Part print with two shaded views. Sizes in mm from the minimum x, y, z corner. A direction names the side the tool comes from. Coordinates: 2 decimals unless noted, no trailing zeros. Order: outer loops, then holes, each group sorted by start corner. A loop starts at its lowest first (then second) coordinate and runs counter-clockwise, first axis right, second up. Notation, with made-up numbers: M -18.5,3.5 L 16.5,3.5 A15 ccw 16.5,32.5 Z; hole C 63.25,20 d7. An arc over 180 degrees is marked long. Answer in a Markdown table with one row per item. Add a question column.
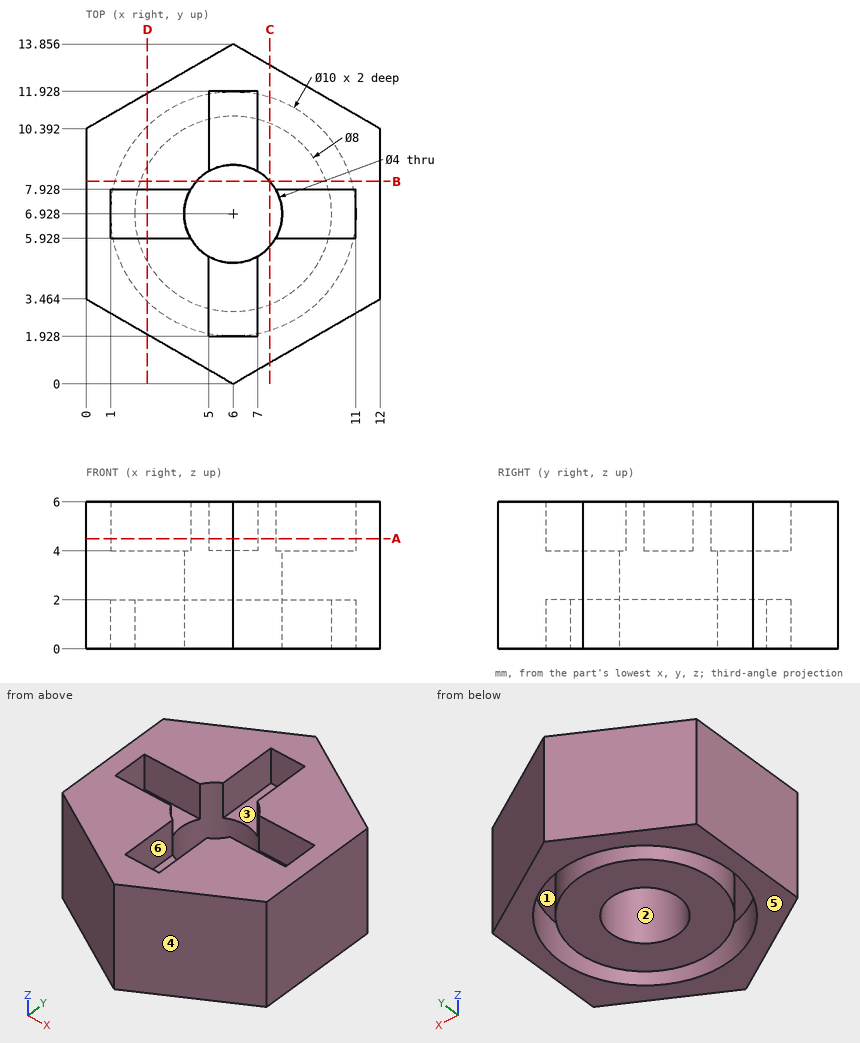
(1) Wall check: line 1 (X direction, y = 10, z = 1.85) (1 decimal); line 2 (X direction, y = 4.75, z = 5.4); line 3 (Z direction, x = 1.5, y = 5). Give the ranges that are in metal, low to high.
(2) 3-axis set-ups, long thin cutter, end or side, ignore diameter. For the marked faces 1, 2 and 3: which of +Z, -Z, +X, -X, +Y, -Y reach the whole face in a straight line?
(3) Slice it at C-C (x = 7.5). List the corners of the cut face in (y, z) (1 decimal).
(4) Slice it at A-A (z = 4.5). List the corners of the cut face in (x, y).
(5) Slice it at B-B (y = 8.25). List the corners of the cut face in (x, z) (1 decimal), and give its area (3 significant figures).
(6) Slice it at D-D (x = 2.5). List the corners of the cut face in (y, z) (1 decimal).
(7) Pull direction Y, two halves, no side cores. Call the marked faces 4, 5 and 6: pulls with the +Y half, pulls with the -Y half, needs draft (parallel to the pull), parting line crosses it, or undercut.
(8) Drop flat-ended pins along their axis: P1, Ø1.5, axis at x = 8, z = 2, coming from the +Y side (1 decimal); P2, Ø0.6, axis at x = 6, y = 3, coming from the +Z side; P3, Ø1, axis at x = 3, z = 5, coming from the -Y side. Give the stop position or say it passes through.
Computed:
| question | item | result |
|---|---|---|
| 1 | line 1 | x = 0 to 2.1, 3.4 to 8.6, 9.9 to 12 |
| 1 | line 2 | x = 0 to 5, 7 to 12 |
| 1 | line 3 | z = 2 to 6 |
| 2 | face 1 | -Z |
| 2 | face 2 | +Z, -Z |
| 2 | face 3 | +Z |
| 3 | outline | M 0.9,0 L 2.2,0 L 2.2,2 L 3.2,2 L 3.2,0 L 5.6,0 L 5.6,6 L 0.9,6 Z; M 8.3,0 L 10.6,0 L 10.6,2 L 11.7,2 L 11.7,0 L 13,0 L 13,6 L 8.3,6 Z |
| 4 | outline | M 0,3.46 L 6,0 L 12,3.46 L 12,10.39 L 6,13.86 L 0,10.39 Z; hole M 1,5.93 L 4.27,5.93 A2 ccw 5,5.2 L 5,1.93 L 7,1.93 L 7,5.2 A2 ccw 7.73,5.93 L 11,5.93 L 11,7.93 L 7.73,7.93 A2 ccw 7,8.66 L 7,11.93 L 5,11.93 L 5,8.66 A2 ccw 4.27,7.93 L 1,7.93 Z |
| 5 | outline | M 0,0 L 1.2,0 L 1.2,2 L 2.2,2 L 2.2,0 L 4.5,0 L 4.5,6 L 0,6 Z; M 7.5,0 L 9.8,0 L 9.8,2 L 10.8,2 L 10.8,0 L 12,0 L 12,6 L 7.5,6 Z |
| 5 | area | 49.8 mm^2 |
| 6 | outline | M 2,0 L 3.4,0 L 3.4,2 L 5,2 L 5,0 L 8.9,0 L 8.9,2 L 10.5,2 L 10.5,0 L 11.8,0 L 11.8,6 L 7.9,6 L 7.9,4 L 5.9,4 L 5.9,6 L 2,6 Z |
| 7 | face 4 | pulls with the -Y half |
| 7 | face 5 | needs draft |
| 7 | face 6 | undercut |
| 8 | P1 | stops at y = 13.1 |
| 8 | P2 | stops at z = 4 |
| 8 | P3 | stops at y = 1.44 |
